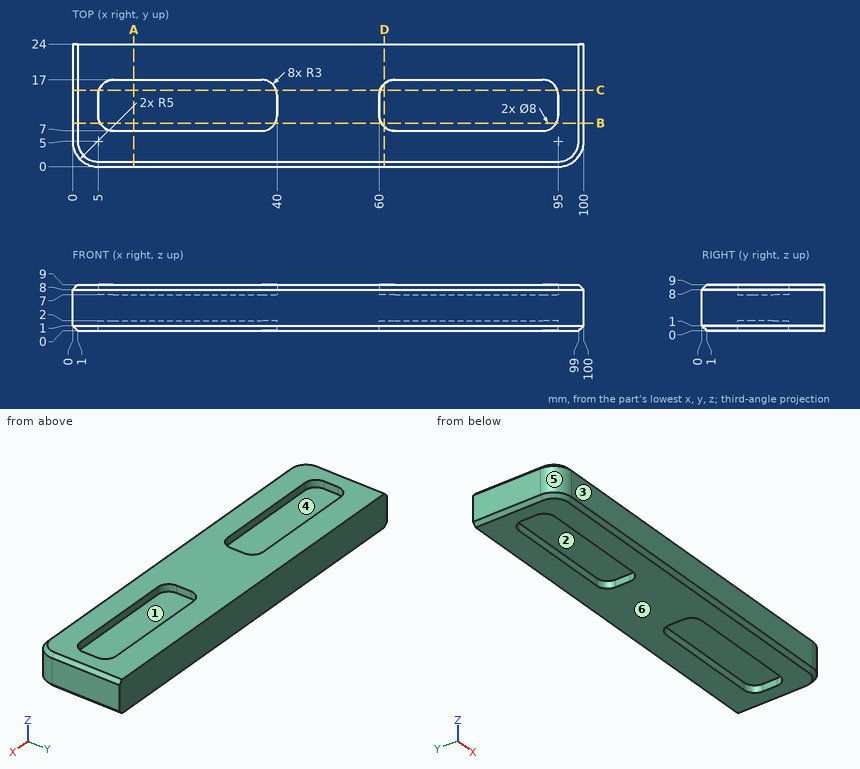
Answer from the drawing. Dimensions are ordinates in mm from the lowest x, y and z of the part. A direction names the side the tool comes from. Give positions to 0.01 mm unless a question says otherwise; leave off trailing zeros. Order: outer loops, then holes, each group sorted by start corner. A loop starts at its lowest first (then second) coordinate and runs counter-clockwise, first axis right, second up. Notation, with made-up numbers: (-28, 35.5) -> (-11, 35.5) arc R18 cw to (-11, 54.5) -> close; hole circle Ø10 at (81.5, 77.25). An arc over 180 degrees is marked (long way). One line per item, written item: value. Start each with the question number.
(1) Straight lines are drawn through the part: L1, parallel to X at y = 8, z = 1; L2, parallel to Z at x = 89, y = 7.5; L3, parallel to X at y = 2, z = 5.25. For each, find the intervals that lie inside material, in ascending order.
(2) The part is cut by section C-C (y = 15). Determine the outline of the cut face in (x, z).
(3) Flat-ended cylindrical pins translate along their axes: P1, Ø5, axis at x = 90, y = 11.5, coming from the -Z side; P2, Ø8, axis at x = 70, y = 13.5, coming from the -Z side. Find the tip coordinate at first contact, or state that the pin passes through.
(4) The part is cut by section B-B (y = 8.5). Determine the outline of the cut face in (x, z).
(5) The part is cut by section A-A (x = 12). Determine the outline of the cut face in (y, z).
(6) A tool of negligible diameter and unlimited length cuts with its end or side. For the marked faces 1, 2 and 3, from which of +Z, -Z, +X, -X, +Y, -Y can it reach the whole face along a straight path? Write none if from no direction.
(7) For a pull along X with two mould halves and no side action, classify the marked faces 4, 5 and 6 as released by +X, released by -X, zero draft, split by the parting line, or undercut.
(8) The part is cut by section D-D (x = 61). Determine the outline of the cut face in (y, z).
Taken from the geometry:
1. L1: 0 to 5.76, 39.24 to 60.76, 94.24 to 100
1. L2: 2 to 7
1. L3: 1 to 99
2. outline: (0, 1) -> (1, 0) -> (5.17, 0) -> (5.17, 2) -> (39.83, 2) -> (39.83, 0) -> (60.17, 0) -> (60.17, 2) -> (94.83, 2) -> (94.83, 0) -> (99, 0) -> (100, 1) -> (100, 8) -> (99, 9) -> (94.83, 9) -> (94.83, 7) -> (60.17, 7) -> (60.17, 9) -> (39.83, 9) -> (39.83, 7) -> (5.17, 7) -> (5.17, 9) -> (1, 9) -> (0, 8) -> close
3. P1: z = 2
3. P2: z = 0
4. outline: (0, 1) -> (1, 0) -> (5.4, 0) -> (5.4, 2) -> (39.6, 2) -> (39.6, 0) -> (60.4, 0) -> (60.4, 2) -> (94.6, 2) -> (94.6, 0) -> (99, 0) -> (100, 1) -> (100, 8) -> (99, 9) -> (94.6, 9) -> (94.6, 7) -> (60.4, 7) -> (60.4, 9) -> (39.6, 9) -> (39.6, 7) -> (5.4, 7) -> (5.4, 9) -> (1, 9) -> (0, 8) -> close
5. outline: (0, 1) -> (1, 0) -> (7, 0) -> (7, 2) -> (17, 2) -> (17, 0) -> (24, 0) -> (24, 9) -> (17, 9) -> (17, 7) -> (7, 7) -> (7, 9) -> (1, 9) -> (0, 8) -> close
6. face 1: +Z
6. face 2: -Z
6. face 3: +Z, -Z, +X, -X, -Y
7. face 4: undercut
7. face 5: released by -X
7. face 6: zero draft
8. outline: (0, 1) -> (1, 0) -> (7.76, 0) -> (7.76, 2) -> (16.24, 2) -> (16.24, 0) -> (24, 0) -> (24, 9) -> (16.24, 9) -> (16.24, 7) -> (7.76, 7) -> (7.76, 9) -> (1, 9) -> (0, 8) -> close
